from build123d import *

# Parameters (mm, degrees)
SKETCH_1_R               = 1.5
EXTRUDE_1_DEPTH          = 10
CUT_EXTRUDE_1_DEPTH      = 52.14684741
CUT_EXTRUDE_1_DEPTH_BACK = 52.14684741
SKETCH_2_R               = 2
SKETCH_2_W               = 10
SKETCH_2_H               = 10
CHAMFER_1_SIZE           = 3


with BuildPart() as part:
    # 草图1 → 凸台-拉伸1 (new, symmetric)
    with BuildSketch(Plane(origin=(0, 0, 0), x_dir=(0, 0, -1), z_dir=(1, 0, 0))):
        with BuildLine():
            Line((0, -4), (-44.803847577, -4))
            Line((-44.803847577, -4), (-50, -1))
            Line((-50, -1), (-50, 0))
            Line((-50, 0), (-4, 0))
            ThreePointArc((-4, 0), (2.828427125, 2.828427125), (0, -4))
        make_face()
        Circle(SKETCH_1_R, mode=Mode.SUBTRACT)
    extrude(amount=EXTRUDE_1_DEPTH, both=True)

    # 草图2 → 切除-拉伸1 (cut, two sides: drawn at the far end of the back side and taken through both)
    with BuildSketch(Plane(origin=(0, 0, 0), x_dir=(1, 0, 0), z_dir=(0, 1, 0)).offset(-CUT_EXTRUDE_1_DEPTH_BACK)):
        with Locations(Location((-5, -20, 0), (0, 0, 270))):
            Circle(SKETCH_2_R)
        with Locations(Location((5, -20, 0), (0, 0, 270))):
            Circle(SKETCH_2_R)
        with Locations((0, -1)):
            Rectangle(SKETCH_2_W, SKETCH_2_H)
    extrude(amount=CUT_EXTRUDE_1_DEPTH + CUT_EXTRUDE_1_DEPTH_BACK, mode=Mode.SUBTRACT)

    # 倒角1
    chamfer_1_edges = [part.edges().sort_by_distance(p)[0] for p in [
        (5, 0, 18),
        (-5, 0, 18),
    ]]
    chamfer(chamfer_1_edges, length=CHAMFER_1_SIZE - 0.0001)  # a hair under: the kernel refuses the full size


solid = part.part
Source: CAD feature listing. Evaluate the final solid. Frame: model axes, mm. A direction names the side the tool comes from. Round coordinates to 2 decimals unless told otherwise and drop trailing zeros. Order: outer loops, then holes, each group sorted by start corner. A loop starts at its lowest first (then second) coordinate and runs counter-clockwise, first axis right, second up. Notation, with made-up numbers: (38, 17) - (91, 17) arc R18 ccw to (91, 48) - close; hole circle Ø2 at (63.5, 59.5). An arc over 180 degrees is marked (long way). Use a Markdown table: item, result. Add a question column.
1. Section query A-A (z = 20). Give the number of separate pieces and of enclosed holes in the cut face, then the cut area to 3 significant figures.
2. Section query D-D (z = 33.5). Return the cut outline in (x, y).
3. First-contact query: pin 1 (4.5 mm diameter, centred on x = 0.5, y = -1, fed in from -Z); pin 2 (6.5 mm diameter, centred on x = -5, z = 20, fed in from -Y); pin 3 (3.5 mm diameter, centred on x = 5, z = 20, fed in from +Y); pin 4 (2 mm diameter, centred on x = -1.5, z = 27.5, fed in from +Y). Flat tips, straight axial feed; report the tip coordinate or a pass-through.
4. Mould query, pull axis Z, two halves, no side actions, for faces 1 (the flat face through (0.1, -0.5, 50)), 2 (the flat face through (0, 0, 27)), 3 (the conical face through (4.34, -2.81, 22.09)). Classes: +Z half, -Z half, draft (parallel to the pull), parting line (faces both ways), or undercut.
5. Section query B-B (y = 2.25). Return the cut outline in (x, z).
6. Set-up query: faces 4 (the cylindrical face through (-7.465, 2.92, -2.734)), 5 (the flat face through (0, -2, 6)). Return all of +Z, -Z, +X, -X, +Y, -Y with unobstructed straight access to the full face (end or side cutting, diameter ignored); none if empty.
7. Line query: probe 1 along X at (y, z) = (-3.4, 20); probe 2 along Y at (x, z) = (-7.7, 0); probe 3 along X at (y, z) = (-3.5, 20.5). Output: solid intervals per line, ascending.
Derived:
| question | item | result |
|---|---|---|
| 1 | separate pieces | 3 |
| 1 | enclosed holes | 0 |
| 1 | area | 30.0 mm2 |
| 2 | outline | (-10, -4) - (10, -4) - (10, 0) - (-10, 0) - close |
| 3 | pin 1 | z = 6 |
| 3 | pin 2 | y = -4 |
| 3 | pin 3 | through |
| 3 | pin 4 | y = 0 |
| 4 | face 1 | +Z half |
| 4 | face 2 | draft |
| 4 | face 3 | undercut |
| 5 | outline | (-10, -3.31) - (-5, -3.31) - (-5, 3.31) - (-10, 3.31) - close; (5, -3.31) - (10, -3.31) - (10, 3.31) - (5, 3.31) - close |
| 6 | face 4 | +X, -X |
| 6 | face 5 | -Z, +Y, -Y |
| 7 | probe 1 | -10 to -7, -3 to 3, 7 to 10 |
| 7 | probe 2 | -4 to -1.5, 1.5 to 4 |
| 7 | probe 3 | -10 to -6.94, -3.06 to 3.06, 6.94 to 10 |
